CAD build for the part. Positions are in the model's coordinates, mm. A direction names the side the tool comes from. Coordinates: 2 decimals unless noted, no trailing zeros. Loops run counter-clockwise (first coordinate to the right, second up) from the corner with the lowest first, then second, coordinate; pieces in that order, holes last. Notation, with made-up numbers: (-39, 65.5) -> (2, 65.5) arc R19 ccw to (2, 85.5) -> close; hole circle Ø4 at (68.5, -16.5). An arc over 180 degrees is marked (long way). Write item = value, one per line. Start each with the question number.
(1) Band-saw the part on D-D (z = -6.5). Write the cut outline in (x, y), and give its area (3 significant figures).
(2) Pull direction X, two halves, no side cores. Call faces 4 (the face through (2.6, 1.97, -12.67)), 5 (the face through (27, 2, 0.176)), 6 (the face through (28.396, 6, -43)): +X half, -X half, draft (parallel to the pull), parting line (faces both ways), or undercut.
(3) Band-saw the part on C-C (x = 10). Write the cut outline in (y, z).
(4) Band-saw the part on A-A (y = 5). Write the cut outline in (x, z) (3 decimals).
(5) Drill centre lines: line 1 (Z direction, x = 27, y = 5); line 2 (Z direction, x = 27.5, y = 3.5); line 3 (Y direction, x = 3, z = -71). Where is each one in solid material? Low to high. Write a range as from..to.
(6) Flat gauge pins, fed straight in: P1, Ø3, axis at y = 4.5, z = -38, coming from the +X side; P2, Ø2, axis at x = 47, y = 1.5, coming from the -Z side; P3, Ø3, axis at y = 6, z = -22.5, coming from the +X side; P4, Ø1.6, axis at x = 7.2, z = -74.92, coming from the -Y side. Where does each tip first touch, or does it go through?
(7) Band-saw the part on B-B (z = -49). Write the cut outline in (x, y), and give its area (3 significant figures).
(8) Tool access for faces 1 (the face through (27, 6, -19.824)), 2 (the face through (25.396, 6, -22)), 3 (the face through (28.396, 6, -64)): list every direction of +Z, -Z, +X, -X, +Y, -Y with a clear straight run to the whole face (end or side of a thin tool).
```python
from build123d import *

# Parameters (mm, degrees)
SKETCH_1_R          = 1
EXTRUDE_2_DEPTH     = 4
SKETCH_3_W          = 3
SKETCH_3_H          = 46
EXTRUDE_3_DEPTH     = 4
SKETCH_4_R          = 1.505
CUT_EXTRUDE_7_DEPTH = 8
CHAMFER_1_SIZE      = 1.5
CHAMFER_2_SIZE      = 1.5


with BuildPart() as part:
    # Эскиз1 → Бобышка-Вытянуть2 (new body)
    with BuildSketch(Plane(origin=(0, 0, 0), x_dir=(1, 0, 0), z_dir=(0, 1, 0))):
        Polygon((2.396260851, 76.824196235), (36.396260851, 76.824196235), (38.396260851, 74.824196235), (53.396260851, 74.824196235), (53.396260851, -0.175803765), (0.396260851, -0.175803765), (0.396260851, 74.824196235), align=None)
        with Locations(Location((7.196260851, 74.924196235, 0), (0, 0, 270))):
            Circle(SKETCH_1_R, mode=Mode.SUBTRACT)
        with Locations(Location((34.196260851, 74.924196235, 0), (0, 0, 270))):
            Circle(SKETCH_1_R, mode=Mode.SUBTRACT)
        with Locations(Location((2.296260851, 13.624196235, 0), (0, 0, 270))):
            Circle(SKETCH_1_R, mode=Mode.SUBTRACT)
        with Locations(Location((48.796260851, 14.624196235, 0), (0, 0, 270))):
            Circle(SKETCH_1_R, mode=Mode.SUBTRACT)
    extrude(amount=EXTRUDE_2_DEPTH)

    # Эскиз3 → Бобышка-Вытянуть3 (add)
    with BuildSketch(Plane(origin=(0, 4, 0), x_dir=(1, 0, 0), z_dir=(0, 1, 0))):
        with Locations((26.896260851, 42.824196235)):
            Rectangle(SKETCH_3_W, SKETCH_3_H)
    extrude(amount=EXTRUDE_3_DEPTH)

    # Эскиз4 → Вырез-Вытянуть7 (cut)
    with BuildSketch(Plane.XZ):
        with Locations(Location((26.896260851, -24.262976388, 0), (0, 0, 270))):
            Circle(SKETCH_4_R)
        with Locations(Location((26.896260851, -62.262976388, 0), (0, 0, 270))):
            Circle(SKETCH_4_R)
    extrude(amount=-CUT_EXTRUDE_7_DEPTH, mode=Mode.SUBTRACT)

    # Фаска1
    chamfer_1_edges = [part.edges().sort_by_distance(p)[0] for p in [
        (26.896260851, 0, -60.757976388),
    ]]
    chamfer(chamfer_1_edges, length=CHAMFER_1_SIZE)

    # Фаска2
    chamfer_2_edges = [part.edges().sort_by_distance(p)[0] for p in [
        (26.896260851, 0, -22.757976388),
    ]]
    chamfer(chamfer_2_edges, length=CHAMFER_2_SIZE)


solid = part.part
```
Findings below:
q1.outline = (0.4, 0) -> (53.4, 0) -> (53.4, 4) -> (0.4, 4) -> close
q1.area = 212 mm²
q2.face_4 = undercut
q2.face_5 = draft
q2.face_6 = +X half
q3.outline = (0, -76.82) -> (4, -76.82) -> (4, 0.18) -> (0, 0.18) -> close
q4.outline = (25.396, -65.824) -> (28.396, -65.824) -> (28.396, -62.386) arc R1.505 cw to (25.396, -62.386) -> close; (25.396, -62.14) arc R1.505 cw to (28.396, -62.14) -> (28.396, -24.386) arc R1.505 cw to (25.396, -24.386) -> close; (25.396, -24.14) arc R1.505 cw to (28.396, -24.14) -> (28.396, -19.824) -> (25.396, -19.824) -> close
q5.line_1 = -65.82..-63.76, -60.76..-25.76, -22.76..-19.82
q5.line_2 = -76.82..-63.64, -60.88..-25.64, -22.88..0.18
q5.line_3 = 0..4
q6.P1 = 53.4
q6.P2 = -74.82
q6.P3 = 28.4
q6.P4 = through
q7.outline = (0.4, 0) -> (53.4, 0) -> (53.4, 4) -> (28.4, 4) -> (28.4, 8) -> (25.4, 8) -> (25.4, 4) -> (0.4, 4) -> close
q7.area = 224 mm²
q8.face_1 = +Z, +X, -X, +Y
q8.face_2 = +Z, -Z, -X, +Y
q8.face_3 = +Z, -Z, +X, +Y
